Here's how the part is built. I have some questions about the finished solid (model axes, mm). Face numbers are marked on the shaded views. A direction names the side the tool comes from. Coordinates: 2 decimals unless noted, no trailing zeros. Order: outer loops, then holes, each group sorted by start corner. A loop starts at its lowest first (then second) coordinate and runs counter-clockwise, first axis right, second up. Notation, with made-up numbers: (-25.75, 40) - (4.25, 40) arc R13 cw to (4.25, 62) - close; hole circle Ø9 at (37, -3.5). An arc over 180 degrees is marked (long way). Answer as CSV lines item,"result". Start each with the question number.
Item 1: On a 3-axis mill with a long thin cutter (end or side, diameter ignored), from which of +Z, -Z, +X, -X, +Y, -Y can I reach the whole of each face in a straight line? I mean the marked faces 1, 2, 3 and 4. Say none if no direction works.
Item 2: I'm going to push flat-ended pins straight in: pin 1 (2 mm diameter, centred on y = -18, z = -16, fed in from -X); pin 2 (3 mm diameter, centred on x = 23.5, y = -24.5, fed in from -Z); pin 3 (8 mm diameter, centred on y = -16, z = -17, fed in from +X); pin 4 (12 mm diameter, centred on x = 30, z = -27.63, fed in from +Y). Where does each tip first touch, or does it pass through?
Item 3: Imagine slicing it at B-B on z = -7. List the corners of the cut face in (x, y) for me, and give its area (3 significant figures).
Item 4: Imagine slicing it at C-C on y = -2. List the corners of the cut face in (x, z) for me, and give its area (3 significant figures).
Item 5: Imagine slicing it at A-A on x = 30. List the corners of the cut face in (y, z) for me, and give its area (3 significant figures).
Item 6: I need wall thicknesses on line 1 (Z direction, x = 22, y = -26.5); line 2 (Y direction, x = 22.5, z = -14); line 3 (X direction, y = -17.25, z = -35). Which ranges of each line are inside material? Lowest first, please.
from build123d import *

# Parameters (mm, degrees)
SKETCH3_W           = 60
SKETCH3_H           = 30
BOSS_EXTRUDE1_DEPTH = 15
SKETCH4_R           = 10
BOSS_EXTRUDE2_DEPTH = 10
FILLET1_R           = 5
FILLET2_R           = 5
FILLET3_R           = 1


with BuildPart() as part:
    # Sketch3 → Boss-Extrude1 (new body)
    with BuildSketch(Plane.XY):
        with Locations((30, -15)):
            Rectangle(SKETCH3_W, SKETCH3_H)
    extrude(amount=BOSS_EXTRUDE1_DEPTH)

    # Sketch4 → Boss-Extrude2 (add, symmetric)
    with BuildSketch(Plane(origin=(0, -15, 0), x_dir=(1, 0, 0), z_dir=(0, 1, 0))):
        with BuildLine():
            Line((10, 27.631533215), (10, 0))
            Line((10, 0), (50, 0))
            Line((50, 0), (50, 27.631533215))
            ThreePointArc((50, 27.631533215), (30, 47.631533215), (10, 27.631533215))
        make_face()
        with Locations(Location((30, 27.631533215, 0), (0, 0, 270))):
            Circle(SKETCH4_R, mode=Mode.SUBTRACT)
    extrude(amount=BOSS_EXTRUDE2_DEPTH, both=True)

    # Fillet1
    fillet1_edges = [part.edges().sort_by_distance(p)[0] for p in [
        (10, -15, 0),
        (50, -15, 0),
    ]]
    fillet(fillet1_edges, radius=FILLET1_R)

    # Fillet2
    # the kernel refuses this fillet: 5 mm, written as the material it takes off along each edge
    with BuildSketch(Plane(origin=(30, -5, -27.631533215), x_dir=(1, 0, 0), z_dir=(0, 0, 1))) as fillet2_piece_1:
        with BuildLine():
            CenterArc((20 - FILLET2_R, -FILLET2_R), FILLET2_R, 0, 90)
            Line((20 - FILLET2_R, 0), (20, 0))
            Line((20, 0), (20, -FILLET2_R))
        make_face()
    revolve(axis=Axis((30, -5, -27.631533215), (0, 1, 0)), revolution_arc=180, mode=Mode.SUBTRACT)
    with BuildSketch(Plane(origin=(10, -5, -27.631533215), x_dir=(0, -1, 0), z_dir=(0, 0, 1)), Plane(origin=(50, -5, -5), x_dir=(0, -1, 0), z_dir=(0, 0, -1))) as fillet2_piece_2:
        with BuildLine():
            CenterArc((FILLET2_R, FILLET2_R), FILLET2_R, 180, 90)
            Line((0, FILLET2_R), (0, 0))
            Line((0, 0), (FILLET2_R, 0))
        make_face()
    extrude(amount=22.631533215, mode=Mode.SUBTRACT)
    with BuildSketch(Plane(origin=(30, -25, -27.631533215), x_dir=(1, 0, 0), z_dir=(0, 0, 1))) as fillet2_piece_3:
        with BuildLine():
            CenterArc((20 - FILLET2_R, FILLET2_R), FILLET2_R, 270, 90)
            Line((20 - FILLET2_R, 0), (20, 0))
            Line((20, 0), (20, FILLET2_R))
        make_face()
    revolve(axis=Axis((30, -25, -27.631533215), (0, 1, 0)), revolution_arc=180, mode=Mode.SUBTRACT)
    with BuildSketch(Plane(origin=(10, -25, -27.631533215), x_dir=(0, 1, 0), z_dir=(0, 0, 1)), Plane(origin=(50, -25, -5), x_dir=(0, 1, 0), z_dir=(0, 0, -1))) as fillet2_piece_4:
        with BuildLine():
            CenterArc((FILLET2_R, -FILLET2_R), FILLET2_R, 90, 90)
            Line((0, -FILLET2_R), (0, 0))
            Line((0, 0), (FILLET2_R, 0))
        make_face()
    extrude(amount=22.631533215, mode=Mode.SUBTRACT)
    with BuildSketch(Plane(origin=(55, -25, -5), x_dir=(0.5976672776328272, 0, -0.8017442392976484), z_dir=(-0.8017442392976484, 0, -0.5976672776328272))) as fillet2_piece_5_section:
        with BuildLine():
            CenterArc((5 + FILLET2_R, -FILLET2_R), FILLET2_R, 90, 90)
            Line((5 + FILLET2_R, 0), (5, 0))
            Line((5, 0), (5, -FILLET2_R))
        make_face()
    fillet2_piece_5 = revolve(axis=Axis((55, -25, -5), (0, -1, 0)), revolution_arc=233.296989237, mode=Mode.PRIVATE)
    fillet2_piece_5 = split(fillet2_piece_5, bisect_by=Plane(origin=(51.250305352, -23.441858441, 0), z_dir=(0, 0, -1)), keep=Keep.TOP, mode=Mode.PRIVATE)
    add(fillet2_piece_5, mode=Mode.SUBTRACT)
    with BuildSketch(Plane(origin=(55, -5, -5), x_dir=(0.5976672776328272, 0, -0.8017442392976484), z_dir=(-0.8017442392976484, 0, -0.5976672776328272))) as fillet2_piece_6_section:
        with BuildLine():
            CenterArc((5 + FILLET2_R, FILLET2_R), FILLET2_R, 180, 90)
            Line((5, FILLET2_R), (5, 0))
            Line((5, 0), (5 + FILLET2_R, 0))
        make_face()
    fillet2_piece_6 = revolve(axis=Axis((55, -5, -5), (0, -1, 0)), revolution_arc=233.296989237, mode=Mode.PRIVATE)
    fillet2_piece_6 = split(fillet2_piece_6, bisect_by=Plane(origin=(51.250305352, -6.558141559, 0), z_dir=(0, 0, -1)), keep=Keep.TOP, mode=Mode.PRIVATE)
    add(fillet2_piece_6, mode=Mode.SUBTRACT)
    with BuildSketch(Plane(origin=(5, -25, -5), x_dir=(-0.5976672776328278, 0, -0.801744239297648), z_dir=(0.801744239297648, 0, -0.5976672776328278))) as fillet2_piece_7_section:
        with BuildLine():
            CenterArc((5 + FILLET2_R, FILLET2_R), FILLET2_R, 180, 90)
            Line((5 + FILLET2_R, 0), (5, 0))
            Line((5, 0), (5, FILLET2_R))
        make_face()
    fillet2_piece_7 = revolve(axis=Axis((5, -25, -5), (0, 1, 0)), revolution_arc=233.296989237, mode=Mode.PRIVATE)
    fillet2_piece_7 = split(fillet2_piece_7, bisect_by=Plane(origin=(8.749694574, -23.441858005, 0), z_dir=(0, 0, -1)), keep=Keep.TOP, mode=Mode.PRIVATE)
    add(fillet2_piece_7, mode=Mode.SUBTRACT)
    with BuildSketch(Plane(origin=(5, -5, -5), x_dir=(-0.5976672776328278, 0, -0.801744239297648), z_dir=(0.801744239297648, 0, -0.5976672776328278))) as fillet2_piece_8_section:
        with BuildLine():
            CenterArc((5 + FILLET2_R, -FILLET2_R), FILLET2_R, 90, 90)
            Line((5 + FILLET2_R, 0), (5, 0))
            Line((5, 0), (5, -FILLET2_R))
        make_face()
    fillet2_piece_8 = revolve(axis=Axis((5, -5, -5), (0, 1, 0)), revolution_arc=233.296989237, mode=Mode.PRIVATE)
    fillet2_piece_8 = split(fillet2_piece_8, bisect_by=Plane(origin=(8.749694574, -6.558141995, 0), z_dir=(0, 0, -1)), keep=Keep.TOP, mode=Mode.PRIVATE)
    add(fillet2_piece_8, mode=Mode.SUBTRACT)

    # Fillet3
    fillet3_edges = [part.edges().sort_by_distance(p)[0] for p in [
        (30, 0, 0),
        (60, -15, 0),
        (30, -30, 0),
        (30, -25, 0),
        (0, -15, 0),
        (30, -5, 0),
        (51.140144071, -23.381125805, 0),
        (8.859855929, -23.381125805, 0),
        (51.140144071, -6.618874195, 0),
        (8.859855929, -6.618874195, 0),
    ]]
    fillet(fillet3_edges, radius=FILLET3_R)


solid = part.part
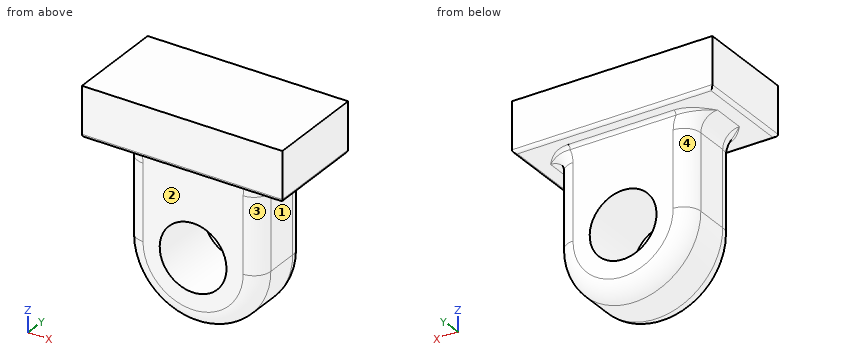
Responses:
1,face 1,"-Z, +X, +Y, -Y"
1,face 2,"-Z, +X, -X, -Y"
1,face 3,"-Z, +X, -Y"
1,face 4,"-Z, -X, +Y"
2,pin 1,"stops at x = 10"
2,pin 2,"stops at z = -45.59"
2,pin 3,"stops at x = 50"
2,pin 4,"passes through"
3,outline,"(10, -20) arc R5 ccw to (15, -25) - (45, -25) arc R5 ccw to (50, -20) - (50, -10) arc R5 ccw to (45, -5) - (15, -5) arc R5 ccw to (10, -10) - close"
3,area,"779 mm^2"
4,outline,"(0, 1) arc R1 ccw to (1, 0) - (59, 0) arc R1 ccw to (60, 1) - (60, 15) - (0, 15) - close"
4,area,"900 mm^2"
5,outline,"(-30, 1) arc R1 ccw to (-29, 0) - (-26, 0) arc R1 cw to (-25, -1) - (-25, -17.63) - (-5, -17.63) - (-5, -1) arc R1 cw to (-4, 0) - (-1, 0) arc R1 ccw to (0, 1) - (0, 15) - (-30, 15) - close; (-25, -42.63) arc R5 ccw to (-20, -47.63) - (-10, -47.63) arc R5 ccw to (-5, -42.63) - (-5, -37.63) - (-25, -37.63) - close"
5,area,"992 mm^2"
6,line 1,"z = 0 to 15"
6,line 2,"y = -25 to -5"
6,line 3,"x = 11.41 to 23.24, 36.76 to 48.59"
